Autodesk Inventor part; units mm, degrees
ref_plane "YZ Plane" through (0, 0, 0) normal (1, 0, 0) x (0, 1, 0)
ref_plane "XZ Plane" through (0, 0, 0) normal (0, 1, 0) x (-1, 0, 0)
ref_plane "XY Plane" through (0, 0, 0) normal (0, 0, 1) x (1, 0, 0)
sketch "Sketch1" plane through (0, 0, 0) normal (0, 1, 0) x (-1, 0, 0)
  line L0 (10, 10) -> (-10, 10)
  line L1 (-10, 10) -> (-10, -10)
  line L2 (-10, -10) -> (10, -10)
  line L3 (10, -10) -> (10, 10)
  line L4 (10, 10) -> (-10, -10) construction
  line L5 (-10, 10) -> (10, -10) construction
  point P0 (0, 0)
  dimension "d0" = 20
  dimension "d1" = 20
extrude "Extrusion1" add sketch "Sketch1" along normal blind 32.5
sketch "Sketch2" plane through (0, 32.5, 0) normal (0, 1, 0) x (1, 0, 0)
  circle A0 centre (0, 0) radius 7.5
  dimension "d4" = 15
extrude "Extrusion2" add sketch "Sketch2" along normal blind 1.6
sketch "Sketch3" plane through (0, 34.1, 0) normal (0, 1, 0) x (1, 0, 0)
  circle A0 centre (0, 0) radius 2
  dimension "d7" = 4
extrude "Extrusion3" add sketch "Sketch3" along normal blind 70
sketch "Sketch5" plane through (0, 34.1, 0) normal (0, 1, 0) x (1, 0, 0)
  circle A0 centre (0, 0) radius 2
  circle A1 centre (0, 0) radius 2.75
  dimension "d10" = 5.5
extrude "Extrusion4" cut sketch "Sketch5" against normal blind 1.6
chamfer "Chamfer1" distance 0.5 angle 45 1 edges at (-2, 104.1, 0)
sketch "Sketch6" plane through (0, 32.5, 0) normal (0, 1, 0) x (1, 0, 0)
  line L0 (-8, -8) -> (8, -8) construction
  line L1 (8, -8) -> (8, 8) construction
  line L2 (8, 8) -> (-8, 8) construction
  line L3 (-8, 8) -> (-8, -8) construction
  line L4 (-8, -8) -> (8, 8) construction
  line L5 (8, -8) -> (-8, 8) construction
  circle A0 centre (-8, 8) radius 1
  circle A1 centre (8, 8) radius 1
  circle A2 centre (8, -8) radius 1
  circle A3 centre (-8, -8) radius 1
  point P0 (0, 0)
  dimension "d16" = 16
  dimension "d17" = 16
  dimension "d18" = 2
  dimension "d19" = 2
  dimension "d20" = 2
  dimension "d21" = 2
extrude "Extrusion5" cut sketch "Sketch6" against normal blind 3
sketch "Sketch7" plane through (0, 0, 0) normal (0, -1, 0) x (1, 0, 0)
  circle A0 centre (0, 0) radius 2.7
  dimension "d24" = 5.4
extrude "Extrusion6" cut sketch "Sketch7" against normal blind 3
sketch "Sketch8" plane through (0, 0, 0) normal (0, -1, 0) x (1, 0, 0)
  line L0 (10, -10) -> (5.5, -10)
  line L1 (5.5, -10) -> (5.5, -5.5)
  line L2 (5.5, -5.5) -> (10, -5.5)
  line L3 (10, -5.5) -> (10, -10)
  line L4 (-10, -10) -> (-5.5, -10)
  line L5 (-5.5, -10) -> (-5.5, -5.5)
  line L6 (-5.5, -5.5) -> (-10, -5.5)
  line L7 (-10, -5.5) -> (-10, -10)
  line L8 (10, 10) -> (10, -10)
  line L9 (10, 10) -> (5.5, 10)
  line L10 (5.5, 10) -> (5.5, 5.5)
  line L11 (5.5, 5.5) -> (10, 5.5)
  line L12 (10, 5.5) -> (10, 10)
  line L13 (-10, 10) -> (10, 10)
  line L14 (-10, 10) -> (-5.5, 10)
  line L15 (-5.5, 10) -> (-5.5, 5.5)
  line L16 (-5.5, 5.5) -> (-10, 5.5)
  line L17 (-10, 5.5) -> (-10, 10)
  line L18 (10, -10) -> (-10, -10)
  point P0 (0, 0)
  dimension "d27" = 11
  dimension "d28" = 11
  dimension "d29" = 5.5
  dimension "d30" = 11
  dimension "d31" = 5.5
  dimension "d32" = 11
extrude "Extrusion7" cut sketch "Sketch8" against normal blind 2
sketch "Sketch9" plane through (0, 2, 0) normal (0, -1, 0) x (1, 0, 0)
  circle A0 centre (8, -8) radius 1.9
  circle A1 centre (-8, -8) radius 1
  circle A2 centre (-8, -8) radius 1.9
  circle A3 centre (-8, 8) radius 1
  circle A4 centre (-8, 8) radius 1.9
  circle A5 centre (8, 8) radius 1
  circle A6 centre (8, 8) radius 1.9
  point P0 (0, 0)
  dimension "d35" = 3.8
  dimension "d36" = 3.8
  dimension "d37" = 3.8
  dimension "d38" = 3.8
extrude "Extrusion8" add sketch "Sketch9" along normal blind 1.6 contours A0 | A1 | A2 | A3 | A4 | A5 | A6
fillet "Fillet1" radius 0.5 4 edges at (-9.9, 0.4, -8) (6.1, 0.4, -8) (6.1, 0.4, 8) (-9.9, 0.4, 8)
fillet "Fillet2" radius 2 4 edges at (-10, 17.25, -10) (10, 17.25, -10) (-10, 17.25, 10) (10, 17.25, 10)
fillet "Fillet3" radius 1 12 edges at (5.5, 1, -10) (-5.5, 1, -5.5) (-5.5, 1, -10) (-10, 1, -5.5) (-10, 1, 5.5) (-5.5, 1, 10) (-5.5, 1, 5.5) (5.5, 1, 10) (5.5, 1, 5.5) (10, 1, 5.5) (5.5, 1, -5.5) (10, 1, -5.5)
thread "Thread1"
properties part number "Nema 8"
Here's how the part is built. I have some questions about the finished solid (model axes, mm). A direction names the side the tool comes from. Give positions to 0.01 mm unless a question says otherwise; leave off trailing zeros. Order: outer loops, then holes, each group sorted by start corner. A loop starts at its lowest first (then second) coordinate and runs counter-clockwise, first axis right, second up. Notation, with made-up numbers: (6.5, 73) -> (56.5, 73) arc R24 cw to (56.5, 105) -> close; hole circle Ø5 at (-25, -24). An arc over 180 degrees is marked (long way). One line per item, written item: value. Start each with the question number.
1. We'd pull the mould along X, two halves only. Please class faces 1 (the face through (-8, 31, -9)), 2 (the face through (8, 1, 5.5)), 3 (the face through (-9.4, 17.46, -9.43)): released by +X, released by -X, zero draft, split by the parting line, or undercut.
2. Imagine slicing it at A-A, the plane z = 0. List the corners of the cut face in (x, y) for me.
3. For faces 4 (the face through (-8, 1, 5.5)), 5 (the face through (6, 2, 7)), 6 (the face through (5.5, 1, -8)), 7 (the face through (5.5, 1, 8)), 8 (the face through (8, 1, -5.5)), which set-ups out of +Z, -Z, +X, -X, +Y, -Y let a thin tool reach every point of the face, with its end or its side?
4. Imagine slicing it at C-C, the plane y = 81. List the corners of the cut face in (x, z) for me.
5. I need wall thicknesses on probe 1 along X at (y, z) = (30.25, 8); probe 2 along X at (y, z) = (33.05, 0). Which ranges of each line are inside material? Lowest first, please. Write a range as from..to.
6. Imagine slicing it at B-B, the plane x = 0. List the corners of the cut face in (y, z) for me, plus the area to 3 significant figures.
7. Will these pins go through, and if not, where does the flat tip stop? pin 1 Ø6 at (x, y) = (1.5, 86) entering from -Z; pin 2 Ø0.6 at (x, z) = (-7.5, 8) entering from +Y; pin 3 Ø3 at (x, z) = (-8, 7.5) entering from -Y.
Values follow:
1. face 1: undercut
1. face 2: zero draft
1. face 3: released by -X
2. outline: (-10, 0) -> (-2.7, 0) -> (-2.7, 3) -> (2.7, 3) -> (2.7, 0) -> (10, 0) -> (10, 32.5) -> (7.5, 32.5) -> (7.5, 34.1) -> (2.75, 34.1) -> (2.75, 32.5) -> (2, 32.5) -> (2, 103.6) -> (1.5, 104.1) -> (-1.5, 104.1) -> (-2, 103.6) -> (-2, 32.5) -> (-2.75, 32.5) -> (-2.75, 34.1) -> (-7.5, 34.1) -> (-7.5, 32.5) -> (-10, 32.5) -> close
3. face 4: -X, -Y
3. face 5: -Y
3. face 6: -Z, -Y
3. face 7: +Z, -Y
3. face 8: +X, -Y
4. outline: circle Ø4 at (0, 0)
5. probe 1: x = -10..-9, -7..7, 9..10
5. probe 2: x = -7.5..-2.75, -2..2, 2.75..7.5
6. outline: (0, -10) -> (32.5, -10) -> (32.5, -7.5) -> (34.1, -7.5) -> (34.1, -2.75) -> (32.5, -2.75) -> (32.5, -2) -> (103.6, -2) -> (104.1, -1.5) -> (104.1, 1.5) -> (103.6, 2) -> (32.5, 2) -> (32.5, 2.75) -> (34.1, 2.75) -> (34.1, 7.5) -> (32.5, 7.5) -> (32.5, 10) -> (0, 10) -> (0, 2.7) -> (3, 2.7) -> (3, -2.7) -> (0, -2.7) -> close
6. area: 935 mm2
7. pin 1: stops at z = -2
7. pin 2: stops at y = 29.5
7. pin 3: stops at y = 0.4
